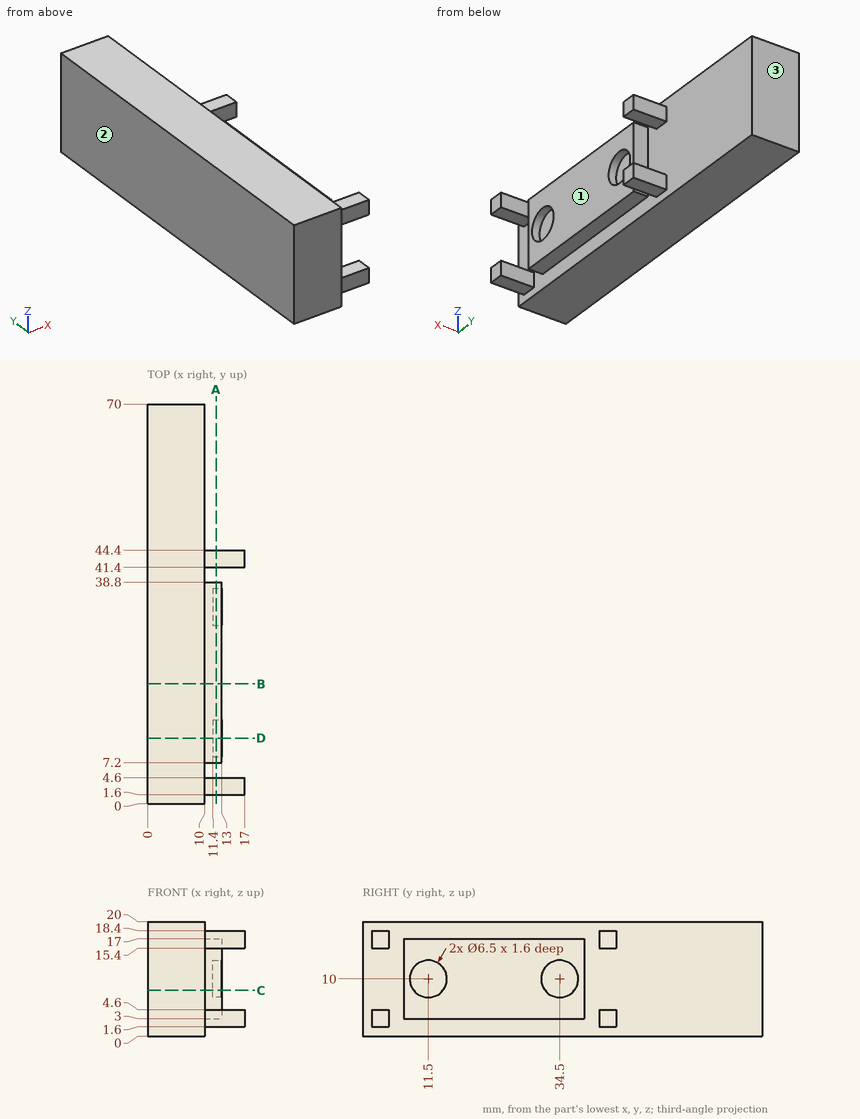
Geometry check sheet. Reference: drawing and pictorial views, mm from the part's lowest x, y, z. Round coordinates to 2 decimals unless told otherwise and drop trailing zeros. Loops run counter-clockwise (first coordinate to the right, second up) from the corner with the lowest first, then second, coordinate; pieces in that order, holes last. Notation, with made-up numbers: (53.25, 22.25) - (90.25, 22.25) arc R23 ccw to (90.25, 38.25) - close; hole circle Ø6 at (-10, 45.5). An arc over 180 degrees is marked (long way). Write item = value, one per line. Start each with the question number.
Q1. Section check D-D (y = 11.5). Record the boundary of the cut face in (x, z).
Q2. Section check A-A (x = 12). Record the boundary of the cut face in (y, z).
Q3. Release check for a two-part mould opening along Y. For the marked faces 1, 2 and 3 record: pulls with the +Y half, pulls with the -Y half, needs draft (parallel to the pull), parting line crosses it, or undercut.
Q4. Section check C-C (z = 8). Record the boundary of the cut face in (x, y).
Q5. Depth check by flat-ended pin: P1, Ø0.9, axis at x = 12, y = 2.5, coming from the +Z side; P2, Ø2.5, axis at x = 11.5, y = 19.5, coming from the -Z side; P3, Ø1.5, axis at x = 11.5, z = 10, coming from the -Y side. Enter the tip coordinate at first touch or a pass-through.
Q6. Thickness scan on L1, parallel to Y at x = 12.3, z = 10; L2, parallel to Y at x = 16, z = 17; L3, parallel to X at y = 67, z = 10.5. Record the ranges inside material, lowest first.
Q7. Section check B-B (y = 21). Record the boundary of the cut face in (x, z), plus the area to 3 significant figures.
Derived:
q1.outline = (0, 0) - (10, 0) - (10, 3) - (13, 3) - (13, 6.75) - (11.4, 6.75) - (11.4, 13.25) - (13, 13.25) - (13, 17) - (10, 17) - (10, 20) - (0, 20) - close
q2.outline = (1.6, 1.6) - (4.6, 1.6) - (4.6, 4.6) - (1.6, 4.6) - close; (1.6, 15.4) - (4.6, 15.4) - (4.6, 18.4) - (1.6, 18.4) - close; (7.2, 3) - (38.8, 3) - (38.8, 17) - (7.2, 17) - close; (41.4, 1.6) - (44.4, 1.6) - (44.4, 4.6) - (41.4, 4.6) - close; (41.4, 15.4) - (44.4, 15.4) - (44.4, 18.4) - (41.4, 18.4) - close; hole circle Ø6.5 at (11.5, 10); hole circle Ø6.5 at (34.5, 10)
q3.face_1 = undercut
q3.face_2 = needs draft
q3.face_3 = pulls with the +Y half
q4.outline = (0, 0) - (10, 0) - (10, 7.2) - (13, 7.2) - (13, 8.94) - (11.4, 8.94) - (11.4, 14.06) - (13, 14.06) - (13, 31.94) - (11.4, 31.94) - (11.4, 37.06) - (13, 37.06) - (13, 38.8) - (10, 38.8) - (10, 70) - (0, 70) - close
q5.P1 = 18.4
q5.P2 = 3
q5.P3 = 7.2
q6.L1 = 7.2 to 8.25, 14.75 to 31.25, 37.75 to 38.8
q6.L2 = 1.6 to 4.6, 41.4 to 44.4
q6.L3 = 0 to 10
q7.outline = (0, 0) - (10, 0) - (10, 3) - (13, 3) - (13, 17) - (10, 17) - (10, 20) - (0, 20) - close
q7.area = 242 mm^2
